Geometry check sheet. Reference: drawing and pictorial views, mm from the part's lowest x, y, z. A direction names the side the tool comes from. Give positions to 0.01 mm unless a question says otherwise; leave off trailing zeros. Order: outer loops, then holes, each group sorted by start corner. A loop starts at its lowest first (then second) coordinate and runs counter-clockwise, first axis right, second up.
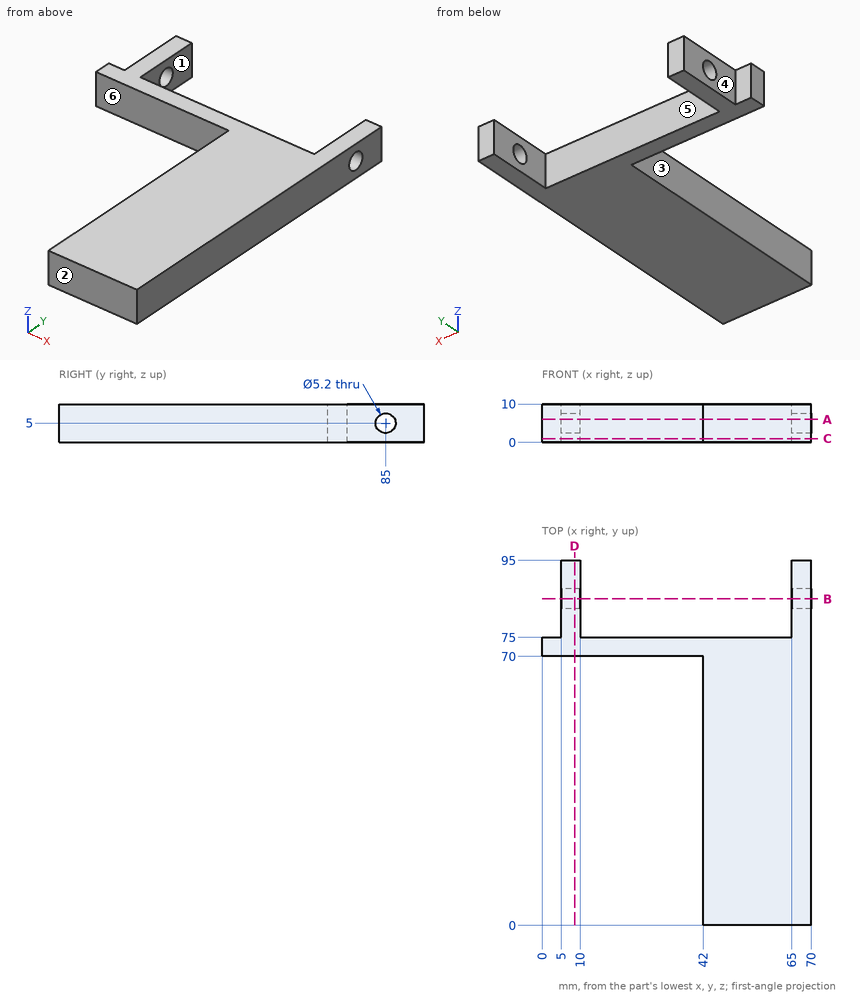
1) Section check D-D, the plane x = 8.5. Record the cut outline in (y, z).
Recorded:
outline: (70, 0) - (95, 0) - (95, 10) - (70, 10) - close; hole circle Ø5.2 at (85, 5)
2) Material ranges on L1, parallel to Y at x = 68.7, z = 5; L2, parallel to X at y = 76, z = 6.5; L3, parallel to Y at x = 7.2, z = 5, recorded low to high.
Recorded:
L1: y = 0 to 82.4, 87.6 to 95
L2: x = 5 to 10, 65 to 70
L3: y = 70 to 82.4, 87.6 to 95
3) Depth check by flat-ended pin: pin 1 Ø1.5 at (x, z) = (3, 7) entering from +Y; pin 2 Ø1.5 at (y, z) = (35, 2.5) entering from -X; pin 3 Ø3 at (y, z) = (85, 5) entering from -X; pin 4 Ø3 at (y, z) = (83, 2.5) entering from -X. Enter the tip coordinate at first touch or a pass-through.
Recorded:
pin 1: stops at y = 75
pin 2: stops at x = 42
pin 3: passes through
pin 4: stops at x = 5
4) Section check C-C, the plane z = 1. Record the cut outline in (x, y).
Recorded:
outline: (0, 70) - (42, 70) - (42, 0) - (70, 0) - (70, 95) - (65, 95) - (65, 75) - (10, 75) - (10, 95) - (5, 95) - (5, 75) - (0, 75) - close
5) Set-up check for the marked faces 4, 5 and 6: record each of +Z, -Z, +X, -X, +Y, -Y from which the full face is reachable in a straight line by a thin tool's end or side.
Recorded:
face 4: +Z, -Z, -X, +Y
face 5: +Z, -Z, +Y
face 6: +Z, -Z, -X, -Y
6) Section check B-B, the plane y = 85. Record the cut outline in (x, z).
Recorded:
outline: (5, 0) - (10, 0) - (10, 2.4) - (5, 2.4) - close; (5, 7.6) - (10, 7.6) - (10, 10) - (5, 10) - close; (65, 0) - (70, 0) - (70, 2.4) - (65, 2.4) - close; (65, 7.6) - (70, 7.6) - (70, 10) - (65, 10) - close
7) Section check A-A, the plane z = 6. Record the cut outline in (x, y), then the cut area to 3 significant figures.
Recorded:
outline: (0, 70) - (42, 70) - (42, 0) - (70, 0) - (70, 82.6) - (65, 82.6) - (65, 75) - (10, 75) - (10, 82.6) - (5, 82.6) - (5, 75) - (0, 75) - close; (5, 87.4) - (10, 87.4) - (10, 95) - (5, 95) - close; (65, 87.4) - (70, 87.4) - (70, 95) - (65, 95) - close
area: 2,460 mm2
8) Draft check along X on the marked faces 1, 2 and 3. Enter one of: +X half, -X half, draft (parallel to the pull), parting line (faces both ways), or undercut.
Recorded:
face 1: undercut
face 2: draft
face 3: -X half
